The drawing under review shows one solid part. Ordinate dimensions are in mm from its lowest x, y, z. A direction names the side the tool comes from. Give positions to 0.01 mm unless a question says otherwise; leave off trailing zeros. Write each loop counter-clockwise with the first axis right and the second up, starting at its lowest first coordinate (ties: lowest second). Pieces come first, ordered by that corner, then holes. Notation, with made-up numbers: M 49,-25 L 78,-25 A25 cw 78,8 Z; hole C 8.25,-9.75 d9. An arc over 180 degrees is marked long. Write each question's results on one line, items separated by ' | '. Start each with the question number.
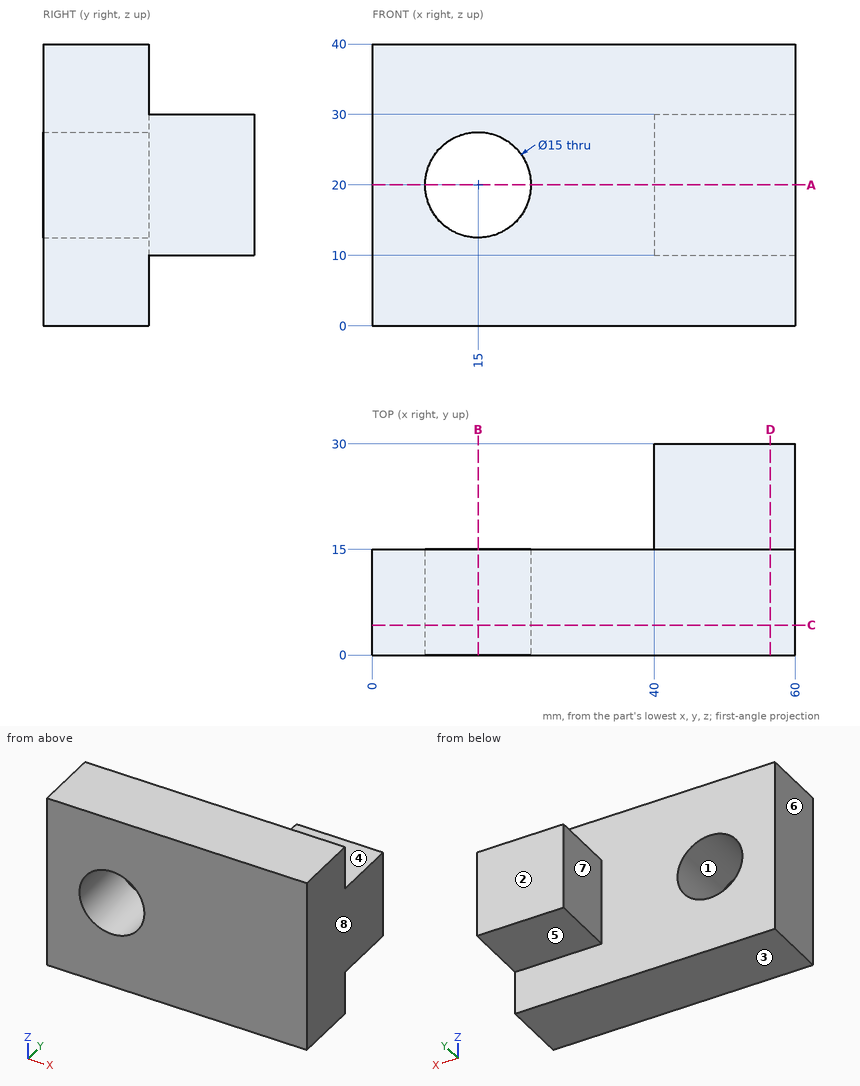
Q1. The part is to be moulded in two halves that separate along Z. For the marked faces 1, 2 and 3, say which applies: pulls with the +Z half, pulls with the -Z half, needs draft (parallel to the pull), parting line crosses it, or undercut.
Q2. For pin 1 Ø4.5 at (x, y) = (46.5, 22.5) entering from -Z; pin 2 Ø1.5 at (x, z) = (25, 24) entering from +Y; pin 3 Ø7.5 at (y, z) = (25.5, 20) entering from -X; pin 4 Ø12 at (x, z) = (15, 20) entering from -Y, all flat-tipped, find the tip position at first contact; note any pin that passes through.
Q3. We need section D-D on x = 56.5. Write out the cut boundary in (y, z), and give its area (3 significant figures).
Q4. For the marked faces 4, 5, 6, 7 and 8, list the 3-axis set-ups (+Z, -Z, +X, -X, +Y, -Y) from which the entire face can be reached by the end or side of a thin tool; tool diameter is ignored.
Q5. We need section B-B on x = 15. Write out the cut boundary in (y, z), and give its area (3 significant figures).
Q6. Wall thickness on line 1 along Z through (x, y) = (15, 6); line 2 along X through (y, z) = (4.75, 20); line 3 along Y through (x, z) = (7, 9): over which ranges is each line inside the solid? List them lowest first. Write a range as from..to.
Q7. We need section C-C on y = 4.25. Write out the cut boundary in (x, z), and give its area (3 significant figures).
Q8. We need section A-A on z = 20. Write out the cut boundary in (x, y), and give its area (3 significant figures).
Answer sheet:
1) face 1: undercut | face 2: needs draft | face 3: pulls with the -Z half
2) pin 1: z = 10 | pin 2: y = 15 | pin 3: x = 40 | pin 4: through
3) outline: M 0,0 L 15,0 L 15,10 L 30,10 L 30,30 L 15,30 L 15,40 L 0,40 Z | area: 900 mm^2
4) face 4: +Z, +X, -X, +Y | face 5: -Z, +X, -X, +Y | face 6: +Z, -Z, -X, +Y, -Y | face 7: +Z, -Z, -X, +Y | face 8: +Z, -Z, +X, +Y, -Y
5) outline: M 0,0 L 15,0 L 15,12.5 L 0,12.5 Z; M 0,27.5 L 15,27.5 L 15,40 L 0,40 Z | area: 375 mm^2
6) line 1: 0..12.5, 27.5..40 | line 2: 0..7.5, 22.5..60 | line 3: 0..15
7) outline: M 0,0 L 60,0 L 60,40 L 0,40 Z; hole C 15,20 d15 | area: 2,220 mm^2
8) outline: M 0,0 L 7.5,0 L 7.5,15 L 0,15 Z; M 22.5,0 L 60,0 L 60,30 L 40,30 L 40,15 L 22.5,15 Z | area: 975 mm^2
